```python
from build123d import *

# Parameters (mm, degrees)
F0_W      = 76.2
F0_H      = 127
F1_DEPTH  = 3.175
F2_W      = 69.85
F2_H      = 120.65
F3_DEPTH  = 3.175
F4_W      = 63.5
F4_H      = 114.3
F5_DEPTH  = 3.175
F6_R      = 3.175
F7_DEPTH  = 56.642
F8_W      = 69.85
F8_H      = 120.65
F9_DEPTH  = 3.175
F9_FACE_W = 69.85
F9_FACE_H = 120.65
F10_DEPTH = 21.59
F12_DEPTH = 123.826


with BuildPart() as f1:
    # F0 (on Top) → F1 (new body)
    with BuildSketch(Plane.XY):
        Rectangle(F0_W, F0_H)
    extrude(amount=F1_DEPTH)

    # F2 (on face) → F3 (join)
    with BuildSketch(Plane.XY.offset(3.175)):
        Rectangle(F2_W, F2_H)
    extrude(amount=F3_DEPTH)

    # F4 (on face) → F5 (join)
    with BuildSketch(Plane.XY.offset(6.35)):
        Rectangle(F4_W, F4_H)
    extrude(amount=F5_DEPTH)

    # F6 (on face) → F7 (join)
    with BuildSketch(Plane.XY.offset(9.525)):
        with Locations((-21.59, 46.99)):
            Circle(F6_R)
        with Locations((-21.59, 31.496)):
            Circle(F6_R)
        with Locations((-21.59, 16.002)):
            Circle(F6_R)
        with Locations((-21.59, 0.508)):
            Circle(F6_R)
        with Locations((-21.59, -14.986)):
            Circle(F6_R)
        with Locations((-21.59, -30.48)):
            Circle(F6_R)
        with Locations((-21.59, -45.974)):
            Circle(F6_R)
        with Locations((-7.366, 46.99)):
            Circle(F6_R)
        with Locations((-7.366, 31.496)):
            Circle(F6_R)
        with Locations((-7.366, 16.002)):
            Circle(F6_R)
        with Locations((-7.366, 0.508)):
            Circle(F6_R)
        with Locations((-7.366, -14.986)):
            Circle(F6_R)
        with Locations((-7.366, -30.48)):
            Circle(F6_R)
        with Locations((-7.366, -45.974)):
            Circle(F6_R)
        with Locations((6.858, 46.99)):
            Circle(F6_R)
        with Locations((6.858, 31.496)):
            Circle(F6_R)
        with Locations((6.858, 16.002)):
            Circle(F6_R)
        with Locations((6.858, 0.508)):
            Circle(F6_R)
        with Locations((6.858, -14.986)):
            Circle(F6_R)
        with Locations((6.858, -30.48)):
            Circle(F6_R)
        with Locations((6.858, -45.974)):
            Circle(F6_R)
        with Locations((21.082, 46.99)):
            Circle(F6_R)
        with Locations((21.082, 31.496)):
            Circle(F6_R)
        with Locations((21.082, 16.002)):
            Circle(F6_R)
        with Locations((21.082, 0.508)):
            Circle(F6_R)
        with Locations((21.082, -14.986)):
            Circle(F6_R)
        with Locations((21.082, -30.48)):
            Circle(F6_R)
        with Locations((21.082, -45.974)):
            Circle(F6_R)
    extrude(amount=F7_DEPTH)

    # F8 (on face) → F9 (join)
    with BuildSketch(Plane.XY.offset(66.167)):
        Rectangle(F8_W, F8_H)
    extrude(amount=F9_DEPTH)

    # F9_face (on face) → F10 (join)
    with BuildSketch(Plane.XY.offset(69.342)):
        Rectangle(F9_FACE_W, F9_FACE_H)
    extrude(amount=F10_DEPTH)

    # F11 (on face) → F12 (cut, through all)
    with BuildSketch(Plane.XZ.offset(60.325)):
        Polygon((34.925, 90.932), (0, 90.932), (34.925, 71.966983), align=None)
        Polygon((-34.925, 71.966983), (0, 90.932), (-34.925, 90.932), align=None)
    extrude(amount=-F12_DEPTH, mode=Mode.SUBTRACT)


solid = f1.part
```
Build history of the part. All positions in model axes, mm. A direction names the side the tool comes from. Round coordinates to 2 decimals unless told otherwise and drop trailing zeros. Loops run counter-clockwise (first coordinate to the right, second up) from the corner with the lowest first, then second, coordinate; pieces in that order, holes last.
Item 1: Drill centre lines: line 1 along Z through (x, y) = (0, 39) (3 decimals); line 2 along X through (y, z) = (-33, 65.5); line 3 along Z through (x, y) = (11.5, -49) (3 decimals). Where is each one in solid material? Low to high.
Item 2: Pin check, flat tips, straight feed: P1, Ø20, axis at x = 16, z = 74.5, coming from the +Y side (3 decimals); P2, Ø3.5, axis at y = -2.5, z = 8, coming from the +X side (3 decimals); P3, Ø3, axis at x = 15.5, y = 12.5, coming from the +Z side. Stop position of each tip, or through.
Item 3: Saw through at A-A (y = 7). List the corners of the cut face in (x, z) (3 decimals), then the cut area to 3 significant figures.
Item 4: Two-plate mould, pull along Z, no slides. Class faces 1 (the face through (0, 60.325, 76)), 2 (the face through (-8.05, 12.9, 37.45)), 3 (the face through (-8.05, -33.58, 37.45)): released by +Z, released by -Z, zero draft, split by the parting line, or undercut.
Item 5: Which spindle directions (+Z, -Z, +X, -X, +Y, -Y) get a long thin tool onto all of the face, cutting with end or side? Do faces 4 (the face through (-18.56, 32.45, 37.45)), 5 (the face through (-34.925, -1, 69)), 6 (the face through (0, -57.15, 8)), 7 (the face through (0, 57.15, 8)). Say none if no direction does.
Item 6: Saw through at B-B (z = 35.5). State how many separate pieces and enclosed holes the cut face has, then the cut area to 3 significant figures.
Worked answers:
1. line 1: z = 0 to 9.525, 66.167 to 90.932
1. line 2: x = -23.52 to -19.66, -9.3 to -5.43, 4.93 to 8.79, 19.15 to 23.01
1. line 3: z = 0 to 9.525, 66.167 to 84.687
2. P1: stops at y = 60.325
2. P2: stops at x = 34.925
2. P3: stops at z = 83.33
3. outline: (-38.1, 0) - (38.1, 0) - (38.1, 3.175) - (34.925, 3.175) - (34.925, 6.35) - (31.75, 6.35) - (31.75, 9.525) - (-31.75, 9.525) - (-31.75, 6.35) - (-34.925, 6.35) - (-34.925, 3.175) - (-38.1, 3.175) - close; (-34.925, 66.167) - (34.925, 66.167) - (34.925, 71.967) - (0, 90.932) - (-34.925, 71.967) - close
3. area: 1,730 mm2
4. face 1: zero draft
4. face 2: undercut
4. face 3: undercut
5. face 4: none
5. face 5: +Z, -X, +Y, -Y
5. face 6: +X, -X, -Y
5. face 7: +X, -X, +Y
6. separate pieces: 28
6. enclosed holes: 0
6. area: 887 mm2
